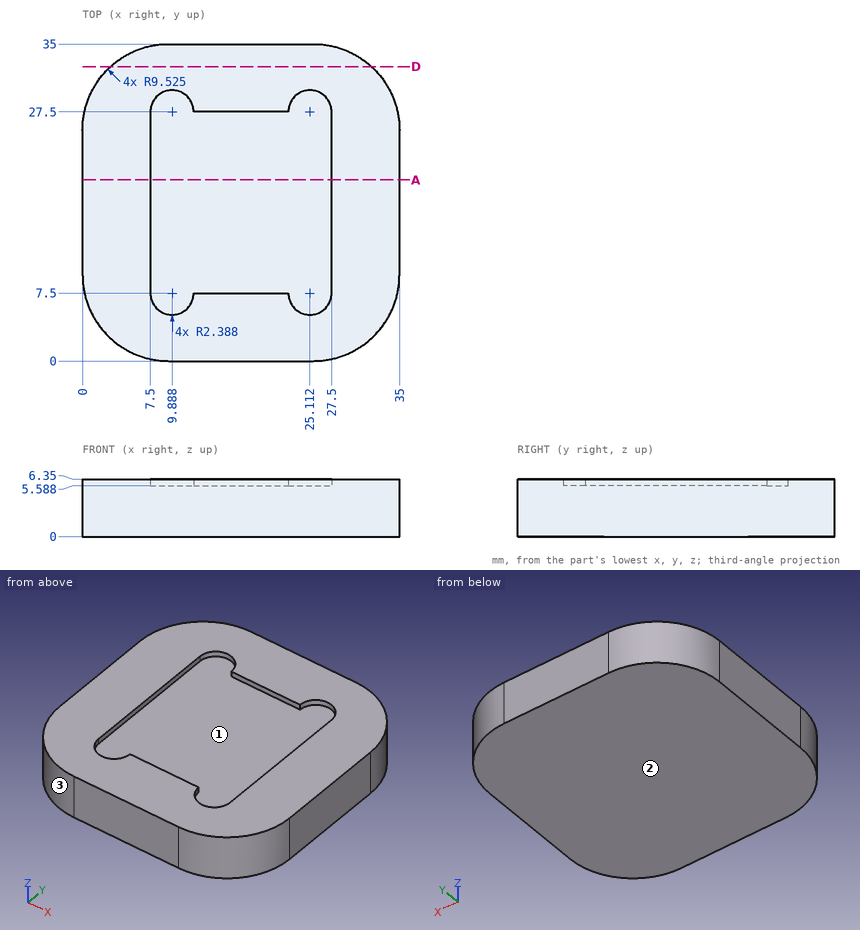
Check sheet for the drawn part. Datum: minimum x, y, z corner. Units: mm. Round coordinates to 2 decimals unless told otherwise and drop trailing zeros. Loops run counter-clockwise (first coordinate to the right, second up) from the corner with the lowest first, then second, coordinate; pieces in that order, holes last.
Item 1: Gauge pin test, flat ends, axial feed: pin 1 (5 mm diameter, centred on x = 22.5, y = 13, fed in from -Z); pin 2 (6 mm diameter, centred on x = 20.5, y = 12, fed in from +Z); pin 3 (2 mm diameter, centred on x = 27.5, z = 3, fed in from +Y) (1 decimal); pin 4 (1 mm diameter, centred on x = 4.5, z = 2, fed in from +Y). Record the tip position at first contact, or that the pin passes through.
Item 2: Mould release check, pull along X, two halves, no side actions. Record for the marked faces 1, 2 and 3: pulls with the +X half, pulls with the -X half, needs draft (parallel to the pull), parting line crosses it, or undercut.
Item 3: Cross-section at D-D on y = 32.5. Record the boundary of the cut face in (x, z), then the cut area to 3 significant figures.
Item 4: Cross-section at A-A on y = 20. Record the boundary of the cut face in (x, z), then the cut area to 3 significant figures.
Item 5: Thickness scan on line 1 (X direction, y = 14.5, z = 6.25); line 2 (Z direction, x = 15.5, y = 24.5); line 3 (Y direction, x = 24, z = 6). Record the ranges inside material, lowest first.
Answer sheet:
1. pin 1: stops at z = 0
1. pin 2: stops at z = 5.59
1. pin 3: stops at y = 34.9
1. pin 4: stops at y = 33.86
2. face 1: undercut
2. face 2: needs draft
2. face 3: pulls with the -X half
3. outline: (3.09, 0) - (31.91, 0) - (31.91, 6.35) - (3.09, 6.35) - close
3. area: 183 mm2
4. outline: (0, 0) - (35, 0) - (35, 6.35) - (27.5, 6.35) - (27.5, 5.59) - (7.5, 5.59) - (7.5, 6.35) - (0, 6.35) - close
4. area: 207 mm2
5. line 1: x = 0 to 7.5, 27.5 to 35
5. line 2: z = 0 to 5.59
5. line 3: y = 0 to 5.39, 29.61 to 35
